from build123d import *

# Parameters (mm, degrees)
BOSS_EXTRUDE1_DEPTH = 10
SKETCH2_R           = 1.6
CUT_EXTRUDE1_DEPTH  = 10
SKETCH3_R           = 3
CUT_EXTRUDE2_DEPTH  = 4


with BuildPart() as part:
    # Sketch1 → Boss-Extrude1 (new body)
    with BuildSketch(Plane.XY):
        Polygon((-5.1, 10), (-5.1, 6), (5.1, 6), (5.1, 10), (30, 10), (30, 0), (-30, 0), (-30, 10), align=None)
    extrude(amount=BOSS_EXTRUDE1_DEPTH)

    # Sketch2 → Cut-Extrude1 (cut)
    with BuildSketch(Plane(origin=(0, 6, 0), x_dir=(1, 0, 0), z_dir=(0, 1, 0))):
        with Locations(Location((0, -5, 0), (0, 0, 270))):
            Circle(SKETCH2_R)
    extrude(amount=-CUT_EXTRUDE1_DEPTH, mode=Mode.SUBTRACT)

    # Sketch3 → Cut-Extrude2 (cut)
    with BuildSketch(Plane.XZ):
        with Locations((0, 5)):
            Circle(SKETCH3_R)
    extrude(amount=-CUT_EXTRUDE2_DEPTH, mode=Mode.SUBTRACT)


solid = part.part
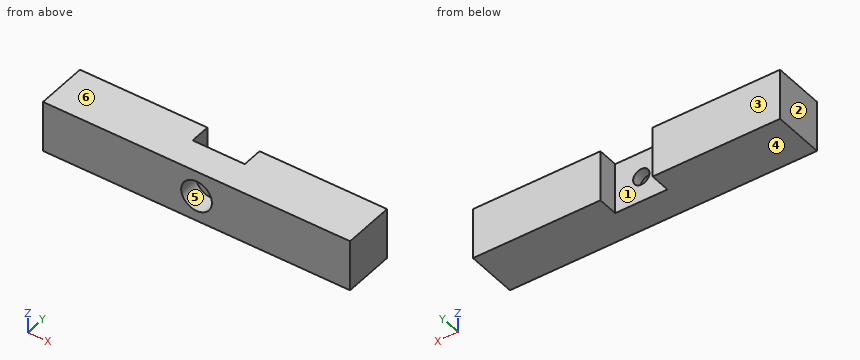
Verification items for the finished model (mm, model axes). Face numbers are marked on the shaded views. A direction names the side the tool comes from. Round coordinates to 2 decimals unless told otherwise and drop trailing zeros. Loops run counter-clockwise (first coordinate to the right, second up) from the corner with the lowest first, then second, coordinate; pieces in that order, holes last. Notation, with made-up numbers: (72, -38) - (103, -38) arc R33 ccw to (103, 1) - close; hole circle Ø1 at (27.25, 19.25). An arc over 180 degrees is marked (long way). Use one line per item in the form item = value.
1. Gauge pin test, flat ends, axial feed: pin 1 Ø5 at (x, y) = (-0.5, 8) entering from +Z; pin 2 Ø5 at (x, z) = (-1, 5) entering from +Y. Record the tip position at first contact, or that the pin passes through.
A:
pin_1 = 10
pin_2 = 6
2. Scan lines: probe 1 along Z at (x, y) = (0, 0.85); probe 2 along X at (y, z) = (4.95, 5); probe 3 along X at (y, z) = (6.25, 4.75). Record each from-to range of solid material in increasing order.
A:
probe_1 = 0 to 2, 8 to 10
probe_2 = -30 to -1.6, 1.6 to 30
probe_3 = -30 to -5.1, 5.1 to 30
3. Section check C-C on y = 1.75. Record the cut outline in (x, z).
A:
outline = (-30, 0) - (30, 0) - (30, 10) - (-30, 10) - close; hole circle Ø6 at (0, 5)
4. Section check D-D on z = 1.25. Record the cut outline in (x, y).
A:
outline = (-30, 0) - (30, 0) - (30, 10) - (5.1, 10) - (5.1, 6) - (-5.1, 6) - (-5.1, 10) - (-30, 10) - close
5. Section check B-B on x = 0. Record the cut outline in (y, z), and give its area (3 significant figures).
A:
outline = (0, 0) - (6, 0) - (6, 3.4) - (4, 3.4) - (4, 2) - (0, 2) - close; (0, 8) - (4, 8) - (4, 6.6) - (6, 6.6) - (6, 10) - (0, 10) - close
area = 29.6 mm²
6. Draft check along Z on the marked faces 3, 4, 5 and 6. Enter one of: pulls with the +Z half, pulls with the -Z half, needs draft (parallel to the pull), parting line crosses it, or undercut.
A:
face_3 = needs draft
face_4 = pulls with the -Z half
face_5 = undercut
face_6 = pulls with the +Z half
7. Section check A-A on z = 5. Record the cut outline in (x, y).
A:
outline = (-30, 0) - (-3, 0) - (-3, 4) - (-1.6, 4) - (-1.6, 6) - (-5.1, 6) - (-5.1, 10) - (-30, 10) - close; (1.6, 4) - (3, 4) - (3, 0) - (30, 0) - (30, 10) - (5.1, 10) - (5.1, 6) - (1.6, 6) - close
8. Access from +Z, -Z, +X, -X, +Y, -Y to the whole of each face (thin tool, end or side, straight path). Record for the marked faces 1 and 2.
A:
face_1 = +Z, -Z, +Y
face_2 = +Z, -Z, -X, +Y, -Y
